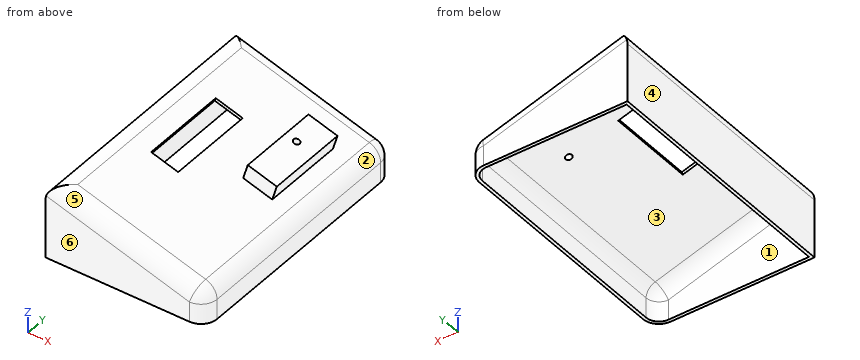
from build123d import *

# Parameters (mm, degrees)
F1_DEPTH = 203.2
F2_R     = 12.7
F3_T     = -2.54
F4_W     = 22.4106954411
F4_H     = 70.1701231301
F5_DEPTH = 25.4
F6_W     = 24.0932293236
F6_H     = 65.9613286316
F7_DEPTH = 12.7
F9_D     = 5.1054


with BuildPart() as f1:
    # F0 (on Front) → F1 (new body)
    with BuildSketch(Plane.XZ):
        Polygon((-1.2532134056, 88.9871907368), (-1.2532134056, 25.4871907368), (125.7467865944, 25.4871907368), (125.7467865944, 50.8871907368), align=None)
    extrude(amount=F1_DEPTH)

    # F2
    f2_edges = [f1.edges().sort_by_distance(p)[0] for p in [
        (-1.253213, -101.6, 88.987191),
        (62.246787, 0, 69.937191),
        (125.746787, -101.6, 50.887191),
        (62.246787, -203.2, 69.937191),
        (125.746787, -203.2, 38.187191),
        (125.746787, 0, 38.187191),
    ]]
    fillet(f2_edges, radius=F2_R)

    # F3
    f3_openings = [f1.faces().sort_by_distance(p)[0] for p in [
        (62.083618, -101.6, 25.487191),
    ]]
    offset(amount=F3_T, openings=f3_openings)

    # F4 (on face) → F5 (cut)
    with BuildSketch(Plane(origin=(24.3884110225, 0, 81.2947034084), x_dir=(0.9578262852, 0, -0.2873478856), z_dir=(0.2873478856, 0, 0.9578262852))):
        with Locations((16.6988200508, -95.6082399935)):
            Rectangle(F4_W, F4_H)
    extrude(amount=-F5_DEPTH, mode=Mode.SUBTRACT)

    # F6 (on face) → F7 (join)
    with BuildSketch(Plane(origin=(24.3884110225, 0, 81.2947034084), x_dir=(0.9578262852, 0, -0.2873478856), z_dir=(0.2873478856, 0, 0.9578262852))):
        with Locations((71.6791953892, -68.6193356842)):
            Rectangle(F6_W, F6_H)
    extrude(amount=F7_DEPTH)

    # F9 (through all)
    with Locations(Plane(origin=(28.0377291692, 0, 93.4590972307), x_dir=(0.9578262852, 0, -0.2873478856), z_dir=(0.2873478856, 0, 0.9578262852))):
        with Locations((68.7415376306, -60.4210160673)):
            Hole(F9_D / 2)


solid = f1.part
Here's how the part is built. I have some questions about the finished solid (model axes, mm). Face numbers are marked on the shaded views. A direction names the side the tool comes from. Coordinates: 2 decimals unless noted, no trailing zeros. Loops run counter-clockwise (first coordinate to the right, second up) from the corner with the lowest first, then second, coordinate; pieces in that order, holes last.
1. For the marked faces 1 and 2, which set-ups out of +Z, -Z, +X, -X, +Y, -Y let a thin tool reach every point of the face, with its end or its side?
2. Imagine slicing it at C-C, the plane y = -149. Please give me the cut outline in (x, z).
3. I need wall thicknesses on L1, parallel to X at y = -74, z = 36; L2, parallel to Y at x = 34.5, z = 60; L3, parallel to Y at x = 86, z = 63. Which ranges of each line are inside material? Lowest first, please.
4. Imagine slicing it at B-B, the plane z = 39. Please give me the cut outline in (x, y).
5. Imagine slicing it at A-A, the plane y = -75. Please give me the cut outline in (x, z).
6. For P1, Ø2.5, axis at x = 36.5, z = 73.5, coming from the +Y side; P2, Ø23, axis at y = -140.5, z = 56, coming from the +X side; P3, Ø5.5, axis at x = 99.5, z = 65, coming from the +Y side, each with a flat end and sliding along its axis, tell me the tip position at first contact or that it passes through.
7. If we mould it in two halves opening along X, with no side actions, what happens to the marked faces 3, 4, 5 and 6? For each: pulls with the +X half, pulls with the -X half, needs draft (parallel to the pull), parting line crosses it, or undercut.
Taken from the geometry:
1. face 1: -Z
1. face 2: +Z, +X, +Y, -Y
2. outline: (-1.25, 25.49) - (1.29, 25.49) - (1.29, 71.92) arc R10.16 cw to (14.37, 81.65) - (115.97, 51.17) arc R10.16 cw to (123.21, 41.44) - (123.21, 25.49) - (125.75, 25.49) - (125.75, 41.44) arc R12.7 ccw to (116.7, 53.6) - (15.1, 84.08) arc R12.7 ccw to (-1.25, 71.92) - close
3. L1: x = -1.25 to 1.29, 123.21 to 125.75
3. L2: y = -203.2 to -200.66, -2.54 to 0
3. L3: y = -101.6 to -35.64
4. outline: (-1.25, -203.2) - (113.05, -203.2) arc R12.7 ccw to (125.75, -190.5) - (125.75, -12.7) arc R12.7 ccw to (113.05, 0) - (-1.25, 0) - close; hole (1.29, -200.66) - (113.05, -200.66) arc R10.16 ccw to (123.21, -190.5) - (123.21, -12.7) arc R10.16 ccw to (113.05, -2.54) - (1.29, -2.54) - close
5. outline: (-1.25, 25.49) - (1.29, 25.49) - (1.29, 71.92) arc R10.16 cw to (14.37, 81.65) - (28.92, 77.28) - (29.65, 79.72) - (15.1, 84.08) arc R12.7 ccw to (-1.25, 71.92) - close; (50.39, 70.84) - (115.97, 51.17) arc R10.16 cw to (123.21, 41.44) - (123.21, 25.49) - (125.75, 25.49) - (125.75, 41.44) arc R12.7 ccw to (116.7, 53.6) - (104.58, 57.24) - (108.23, 69.4) - (85.16, 76.32) - (81.51, 64.16) - (51.12, 73.28) - close
6. P1: stops at y = -2.43
6. P2: stops at x = 125.37
6. P3: stops at y = -35.64
7. face 3: undercut
7. face 4: pulls with the -X half
7. face 5: pulls with the +X half
7. face 6: needs draft
